The model under review builds one solid part; all positions refer to its coordinate system, in mm. A direction names the side the tool comes from. Round coordinates to 2 decimals unless told otherwise and drop trailing zeros. Order: outer loops, then holes, each group sorted by start corner. A loop starts at its lowest first (then second) coordinate and runs counter-clockwise, first axis right, second up. Notation, with made-up numbers: M 43.25,43.5 L 58.25,43.5 A18 ccw 58.25,72.5 Z; hole C 48,34.5 d6. An arc over 180 degrees is marked long. Use a Markdown table: item, result. Add a question column.
1. The part is to be moulded in two halves that separate along Y. For faces 4 (the cylindrical face through (-0.738, 2.345, 6.422)), 5 (the flat face through (-1.4, 3.1, 0)), 6 (the cylindrical face through (3.464, 1.436, 7.789)), say which applies: +Y half, -Y half, draft (parallel to the pull), parting line (faces both ways), or undercut.
2. Consider section D-D on x = 3. State the section outline as (y, z) points, then the cut area to 3 significant figures.
3. For faces 1 (the flat face through (-0.1, -2.3, 15.8)), 2 (the flat face through (2, 2, 3)), 3 (the flat face through (-3, 0, 14.8)), list the 3-axis set-ups (+Z, -Z, +X, -X, +Y, -Y) from which the entire face can be reached by the end or side of a thin tool; tool diameter is ignored.
4. Consider section C-C on y = -3. State the section outline as (x, z) points, then the cut area to 3 significant figures.
5. To check wall thickness, follow probe 1 along Y at (x, z) = (0, 1.7); probe 2 along X at (y, z) = (0, 13.75); probe 3 along X at (y, z) = (0, 4.75). State the ranges of each line that lie inside material, in increasing order.
6. Consider section B-B on y = -1.75. State the section outline as (x, z) points, then the cut area to 3 significant figures.
7. Consider section A-A on x = 0. State the section outline as (y, z) points, then the cut area to 3 significant figures.
8. Insertion check: P1, Ø4, axis at y = 2.5, z = 13.5, coming from the -X side; P2, Ø1.1, axis at x = -3, z = 15.5, coming from the -Y side; P3, Ø2, axis at y = 2, z = 2.5, coming from the +X side; P4, Ø3, axis at x = 0, y = 0, coming from the +Z side. Each pin has a flat end and moves straight along its axis. Give the tip position at first contact, or say it passes through.
Autodesk Inventor part; units mm, degrees
ref_plane "YZ Plane" through (0, 0, 0) normal (1, 0, 0) x (0, 1, 0)
ref_plane "XZ Plane" through (0, 0, 0) normal (0, 1, 0) x (-1, 0, 0)
ref_plane "XY Plane" through (0, 0, 0) normal (0, 0, 1) x (1, 0, 0)
sketch "Sketch1" plane through (0, 0, 0) normal (0, 0, 1) x (1, 0, 0)
  circle A0 centre (0, 0) radius 3.75
  dimension "d0" = 7.5
extrude "Extrusion1" add sketch "Sketch1" along normal blind 15.8
sketch "Sketch2" plane through (0, 0, 0) normal (0, 0, -1) x (-1, 0, 0)
  circle A0 centre (0, 0) radius 3.75
  circle A1 centre (0, 0) radius 3.25
  dimension "d3" = 6.5
extrude "Extrusion2" cut sketch "Sketch2" against normal blind 3 contours A1
hole "Hole1" at (0, 0, 3) direction (0, 0, 1) diameter 4.917 depth 6.75
hole "Hole2" at (0, 0, 15.8) direction (0, 0, -1) diameter 4 end through all
sketch "Sketch3" plane through (0, 0, 0) normal (1, 0, 0) x (0, 1, 0)
  line L0 (-2, 15.8) -> (2, 15.8)
  line L1 (0.8, 15.8) -> (-0.8, 15.8)
  line L2 (-0.8, 15.8) -> (-0.8, 14.8)
  line L3 (-0.8, 14.8) -> (0.8, 14.8)
  line L4 (0.8, 14.8) -> (0.8, 15.8)
  point P0 (0, 0)
  point P1 (0, 15.8)
  dimension "d26" = 1.6
  dimension "d27" = 1
extrude "Extrusion3" cut sketch "Sketch3" along normal through all both and the other way through all
properties part number "308-10" material "PC/ABS Plastic"
Answer block:
| question | item | result |
|---|---|---|
| 1 | face 4 | undercut |
| 1 | face 5 | draft |
| 1 | face 6 | parting line |
| 2 | outline | M -2.25,0 L -1.25,0 L -1.25,3 L 1.25,3 L 1.25,0 L 2.25,0 L 2.25,15.8 L 0.8,15.8 L 0.8,14.8 L -0.8,14.8 L -0.8,15.8 L -2.25,15.8 Z |
| 2 | area | 62.0 mm^2 |
| 3 | face 1 | +Z, +X, -X, +Y, -Y |
| 3 | face 2 | -Z |
| 3 | face 3 | +Z, +X, -X |
| 4 | outline | M -2.25,0 L -1.25,0 L -1.25,3 L 1.25,3 L 1.25,0 L 2.25,0 L 2.25,15.8 L -2.25,15.8 Z |
| 4 | area | 63.6 mm^2 |
| 5 | probe 1 | -3.75 to -3.25, 3.25 to 3.75 |
| 5 | probe 2 | -3.75 to -2, 2 to 3.75 |
| 5 | probe 3 | -3.75 to -2.46, 2.46 to 3.75 |
| 6 | outline | M -3.32,0 L -2.74,0 L -2.74,3 L -1.73,3 L -1.73,9.75 L -0.97,9.75 L -0.97,15.8 L -3.32,15.8 Z; M 0.97,9.75 L 1.73,9.75 L 1.73,3 L 2.74,3 L 2.74,0 L 3.32,0 L 3.32,15.8 L 0.97,15.8 Z |
| 6 | area | 53.3 mm^2 |
| 7 | outline | M -3.75,0 L -3.25,0 L -3.25,3 L -2.46,3 L -2.46,9.75 L -2,9.75 L -2,15.8 L -3.75,15.8 Z; M 2,9.75 L 2.46,9.75 L 2.46,3 L 3.25,3 L 3.25,0 L 3.75,0 L 3.75,15.8 L 2,15.8 Z |
| 7 | area | 41.6 mm^2 |
| 8 | P1 | x = -3.72 |
| 8 | P2 | y = -2.84 |
| 8 | P3 | x = 3.61 |
| 8 | P4 | through |
